Geometry check sheet. Reference: the model listing, model coordinates, mm. Round coordinates to 2 decimals unless told otherwise and drop trailing zeros.
(1) Cross-section at A-A on z = 211.5. Count the separate pieces of the cut face and the enclosed holes in it, and give its area (3 significant figures).
(2) Thickness scan on L1, parallel to Y at x = 3.5, z = 166.5; L2, parallel to Y at x = 5, z = 760; L3, parallel to Y at x = -10.1, z = 433. Record the ranges inside material, lowest first.
(3) Gauge pin test, flat end, axial feed: P1, Ø6, axis at y = 0, z = 258, coming from the +X side. Record the tip position at first contact, or that the pin passes through.
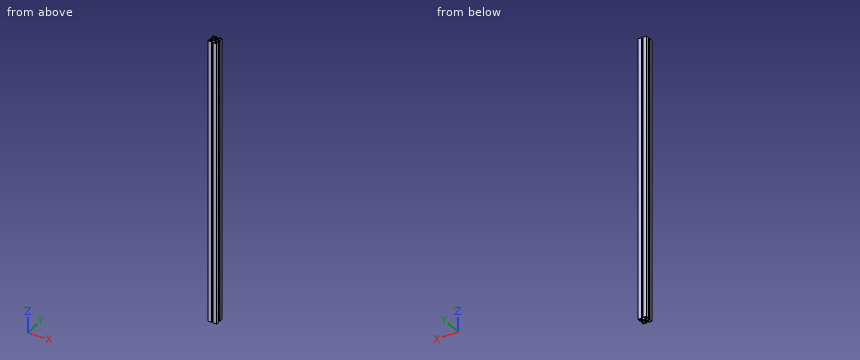
from build123d import *

# Parameters (mm, degrees)
SKETCH_1_R      = 3.5
SKETCH_1_R_2    = 2.5
EXTRUDE_1_DEPTH = 1000


with BuildPart() as part:
    # Эскиз1 → Бобышка-Вытянуть1 (new body)
    with BuildSketch(Plane.XY):
        with BuildLine():
            Line((-15, 5.2), (-15, 15))
            Line((-15, 15), (-5.2, 15))
            Line((-5.2, 15), (-3.25, 15))
            Line((-3.25, 15), (-3.25, 12.8))
            Line((-3.25, 12.8), (-5.2, 12.8))
            Line((-5.2, 12.8), (-5.2, 6.8))
            ThreePointArc((-5.2, 6.8), (0, 4.2), (5.2, 6.8))
            Line((5.2, 6.8), (5.2, 12.8))
            Line((5.2, 12.8), (3.25, 12.8))
            Line((3.25, 12.8), (3.25, 15))
            Line((3.25, 15), (5.2, 15))
            Line((5.2, 15), (15, 15))
            Line((15, 15), (15, 5.2))
            Line((15, 5.2), (15, 3.25))
            Line((15, 3.25), (12.8, 3.25))
            Line((12.8, 3.25), (12.8, 5.2))
            Line((12.8, 5.2), (6.8, 5.2))
            ThreePointArc((6.8, 5.2), (4.2, 0), (6.8, -5.2))
            Line((6.8, -5.2), (12.8, -5.2))
            Line((12.8, -5.2), (12.8, -3.25))
            Line((12.8, -3.25), (15, -3.25))
            Line((15, -3.25), (15, -5.2))
            Line((15, -5.2), (15, -15))
            Line((15, -15), (5.2, -15))
            Line((5.2, -15), (3.25, -15))
            Line((3.25, -15), (3.25, -12.8))
            Line((3.25, -12.8), (5.2, -12.8))
            Line((5.2, -12.8), (5.2, -6.8))
            ThreePointArc((5.2, -6.8), (0, -4.2), (-5.2, -6.8))
            Line((-5.2, -6.8), (-5.2, -12.8))
            Line((-5.2, -12.8), (-3.25, -12.8))
            Line((-3.25, -12.8), (-3.25, -15))
            Line((-3.25, -15), (-5.2, -15))
            Line((-5.2, -15), (-15, -15))
            Line((-15, -15), (-15, -5.2))
            Line((-15, -5.2), (-15, -3.25))
            Line((-15, -3.25), (-12.8, -3.25))
            Line((-12.8, -3.25), (-12.8, -5.2))
            Line((-12.8, -5.2), (-6.8, -5.2))
            ThreePointArc((-6.8, -5.2), (-4.2, 0), (-6.8, 5.2))
            Line((-6.8, 5.2), (-12.8, 5.2))
            Line((-12.8, 5.2), (-12.8, 3.25))
            Line((-12.8, 3.25), (-15, 3.25))
            Line((-15, 3.25), (-15, 5.2))
        make_face()
        with Locations((-10.1, 10.1)):
            Circle(SKETCH_1_R, mode=Mode.SUBTRACT)
        with Locations((10.1, 10.1)):
            Circle(SKETCH_1_R, mode=Mode.SUBTRACT)
        with Locations((-10.1, -10.1)):
            Circle(SKETCH_1_R, mode=Mode.SUBTRACT)
        with Locations((10.1, -10.1)):
            Circle(SKETCH_1_R, mode=Mode.SUBTRACT)
        Circle(SKETCH_1_R_2, mode=Mode.SUBTRACT)
    extrude(amount=EXTRUDE_1_DEPTH)


solid = part.part
Found:
1. separate pieces: 1
1. enclosed holes: 5
1. area: 344 mm2
2. L1: y = -15 to -12.8, -5.22 to 5.22, 12.8 to 15
2. L2: y = -15 to -12.8, -6.55 to -3.12, 3.12 to 6.55, 12.8 to 15
2. L3: y = -15 to -13.6, -6.6 to -5.2, 5.2 to 6.6, 13.6 to 15
3. P1: stops at x = 4.93
